Job drawing, mm, ordinate dimensions from the low corner. One solid piece. Give positions to 0.01 mm unless a question says otherwise; leave off trailing zeros. Order: outer loops, then holes, each group sorted by start corner. A loop starts at its lowest first (then second) coordinate and runs counter-clockwise, first axis right, second up.
Item 1: Band-saw the part on A-A on x = 241.3. Give the cut face in (y, z), plus the area to 3 significant figures.
Item 2: Flat gauge pins, fed straight in: P1, Ø10.5, axis at x = 12.7, y = 190.5, coming from the +Z side; P2, Ø12, axis at x = 92, y = 151.5, coming from the -Z side. Where does each tip first touch, or does it go through?
Item 3: Band-saw the part on B-B on x = 127. Give the cut face in (y, z), plus the area to 3 significant figures.
Item 4: Band-saw the part on D-D on y = 101.6. Give the cut face in (x, z), plus the area to 3 significant figures.
Item 5: Band-saw the part on C-C on y = 190.5. Give the cut face in (x, z), plus the area to 3 significant figures.
Item 6: Wall check: L1, parallel to Y at x = 127, z = 1.95; L2, parallel to Y at x = 12.7, z = 3.9; L3, parallel to X at y = 184.5, z = 1.55. Give the ranges that are in metal, low to high.
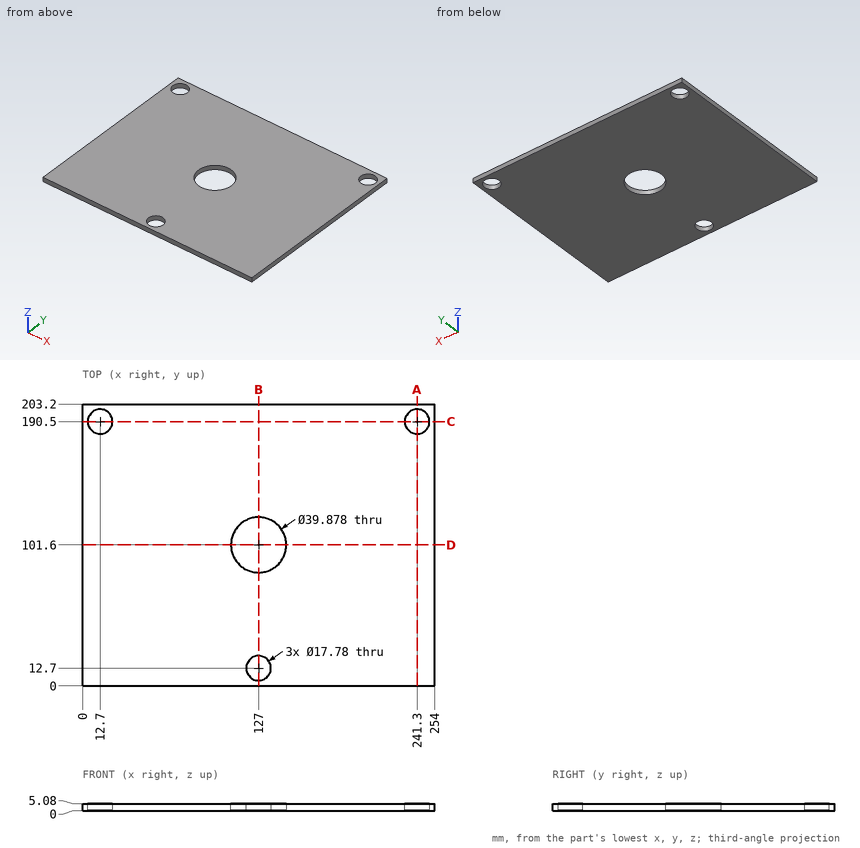
The answers:
1. outline: (0, 0) - (181.61, 0) - (181.61, 5.08) - (0, 5.08) - close; (199.39, 0) - (203.2, 0) - (203.2, 5.08) - (199.39, 5.08) - close
1. area: 942 mm2
2. P1: passes through
2. P2: stops at z = 0
3. outline: (0, 0) - (3.81, 0) - (3.81, 5.08) - (0, 5.08) - close; (21.59, 0) - (81.66, 0) - (81.66, 5.08) - (21.59, 5.08) - close; (121.54, 0) - (203.2, 0) - (203.2, 5.08) - (121.54, 5.08) - close
3. area: 739 mm2
4. outline: (0, 0) - (107.06, 0) - (107.06, 5.08) - (0, 5.08) - close; (146.94, 0) - (254, 0) - (254, 5.08) - (146.94, 5.08) - close
4. area: 1,090 mm2
5. outline: (0, 0) - (3.81, 0) - (3.81, 5.08) - (0, 5.08) - close; (21.59, 0) - (232.41, 0) - (232.41, 5.08) - (21.59, 5.08) - close; (250.19, 0) - (254, 0) - (254, 5.08) - (250.19, 5.08) - close
5. area: 1,110 mm2
6. L1: y = 0 to 3.81, 21.59 to 81.66, 121.54 to 203.2
6. L2: y = 0 to 181.61, 199.39 to 203.2
6. L3: x = 0 to 6.14, 19.26 to 234.74, 247.86 to 254
